Source: CAD feature listing. Evaluate the final solid. Frame: model axes, mm. A direction names the side the tool comes from. Round coordinates to 2 decimals unless told otherwise and drop trailing zeros. Loops run counter-clockwise (first coordinate to the right, second up) from the corner with the lowest first, then second, coordinate; pieces in that order, holes last. Notation, with made-up numbers: (-17, 12.25) -> (28, 12.25) arc R17 ccw to (28, 40.25) -> close; hole circle Ø9 at (42, -3.75). An arc over 180 degrees is marked (long way). Return JSON: item names as keys, results as strings. Group by question number.
```python
from build123d import *

# Parameters (mm, degrees)
F1_DEPTH    = 38.1
F2_R        = 1.778
F3_R        = 5.08
F4_R        = 1.016
F5_DEPTH    = 25.4
F6_T1_DEPTH = 28.575


# Not quite as in the source:
# - a fillet or chamfer that OpenCascade refuses, or shapes differently, is made with other operations: its cross-section is extruded or revolved along the edge and cut away or added


with BuildPart() as f1:
    # F0 (on Front) → F1 (new body)
    with BuildSketch(Plane.XZ):
        Polygon((0, 5.715), (0, 0), (19.05, 0), (19.05, 1.27), (11.1125, 1.27), (11.1125, 10.16), (7.9375, 10.16), (7.9375, 5.715), align=None)
    extrude(amount=F1_DEPTH)

    # F2
    f2_edges = [f1.edges().sort_by_distance(p)[0] for p in [
        (7.9375, -19.05, 5.715),
    ]]
    fillet(f2_edges, radius=F2_R)

    # F3
    f3_edges = [f1.edges().sort_by_distance(p)[0] for p in [
        (19.05, -38.1, 0.635),
        (0, -38.1, 2.8575),
        (0, 0, 2.8575),
        (19.05, 0, 0.635),
    ]]
    fillet(f3_edges, radius=F3_R)

    # F4 (on face) → F5 (cut)
    with BuildSketch(Plane.XY.offset(1.27)):
        with Locations((14.9681093171, -19.05)):
            Circle(F4_R)
    extrude(amount=-F5_DEPTH, mode=Mode.SUBTRACT)

    # F6: fillet of radius 5.08 on 2 edges, made by hand

    # F6_s2 → F6_t1 (cut)
    with BuildSketch(Plane.YZ.offset(-4.7625)):
        with BuildLine():
            ThreePointArc((-33.02, 10.16), (-36.6121024484, 8.6721024484), (-38.1, 5.08))
            Line((-38.1, 5.08), (-38.1, 10.16))
            Line((-38.1, 10.16), (-33.02, 10.16))
        make_face()
        with BuildLine():
            ThreePointArc((0, 5.08), (-1.4878975516, 8.6721024484), (-5.08, 10.16))
            Line((-5.08, 10.16), (0, 10.16))
            Line((0, 10.16), (0, 5.08))
        make_face()
    extrude(amount=F6_T1_DEPTH, mode=Mode.SUBTRACT)


solid = f1.part
```
(1) Cut plane D-D (z = 3). Return loops of the section in (x, y).
(2) Set-up query: faces 4 (the face through (3, -19, 5.715)), 5 (the face through (13, -19, 1.27)), 6 (the face through (19.05, -19, 1)). Return all of +Z, -Z, +X, -X, +Y, -Y with unobstructed straight access to the full face (end or side cutting, diameter ignored); none if empty.
(3) Cut plane B-B (x = 15). Return loops of the section in (y, z).
(4) Ray query, line 1 (X direction, y = -7.5, z = 3.5); line 2 (Z direction, x = 17.5, y = -29); line 3 (Y direction, x = 10.25, z = 6.5). Return the intervals inside material, ascending.
(5) Pin query (flat end, axial travel): pin 1 (3 mm diameter, centred on x = 3.5, y = -12, fed in from +Z) (3 decimals); pin 2 (5 mm diameter, centred on y = -13.5, z = 8, fed in from +X); pin 3 (4 mm diameter, centred on y = -12.5, z = 1.5, fed in from +X); pin 4 (1.3 mm diameter, centred on y = -19, z = 8, fed in from -X). Return the tip coordinate at first contact, or that it passes through.
(6) Mould query, pull axis Y, two halves, no side actions, for faces 1 (the face through (17.522, -1.449, 0.644)), 2 (the face through (15.907, -19.439, 0.644)), 3 (the face through (8, -38.1, 3)). Classes: released by +Y, released by -Y, zero draft, split by the parting line, or undercut.
Answers follow:
{
 "1": {"outline": "(0, -33.02) arc R5.08 ccw to (5.08, -38.1) -> (11.11, -38.1) -> (11.11, 0) -> (5.08, 0) arc R5.08 ccw to (0, -5.08) -> close"},
 "2": {"face 4": "+Z, -X, +Y, -Y", "face 5": "+Z, +X, +Y, -Y", "face 6": "+Z, -Z, +X, +Y, -Y"},
 "3": {"outline": "(-37.99, 0) -> (-20.07, 0) -> (-20.07, 1.27) -> (-37.99, 1.27) -> close; (-18.03, 0) -> (-0.11, 0) -> (-0.11, 1.27) -> (-18.03, 1.27) -> close"},
 "4": {"line 1": "0 to 11.11", "line 2": "0 to 1.27", "line 3": "-37.9 to -0.2"},
 "5": {"pin 1": "z = 5.715", "pin 2": "x = 11.11", "pin 3": "x = 19.05", "pin 4": "x = 7.93"},
 "6": {"face 1": "released by +Y", "face 2": "undercut", "face 3": "released by -Y"}
}
